The model under review builds one solid part; all positions refer to its coordinate system, in mm. A direction names the side the tool comes from. Round coordinates to 2 decimals unless told otherwise and drop trailing zeros. Loops run counter-clockwise (first coordinate to the right, second up) from the corner with the lowest first, then second, coordinate; pieces in that order, holes last. Notation, with made-up numbers: (74.25, -17.75) -> (94.25, -17.75) arc R20 ccw to (94.25, 21.25) -> close; hole circle Ø10 at (-1, -31.75). An arc over 180 degrees is marked (long way). Use a Markdown table: item, result. Add a question column.
1) Insertion check: pin 1 (1 mm diameter, centred on y = 5.5, z = -20, fed in from +X); pin 2 (4 mm diameter, centred on x = 8, y = 5.5, fed in from +Z); pin 3 (2.5 mm diameter, centred on x = -14.5, y = 4.5, fed in from -Z). Each pin has a flat end and moves straight along its axis. Give the tip position at first contact, or say it passes through.
2) Consider section A-A on x = 56. Give the boundary of the cut face in (y, z).
3) Mouldability with a two-part tool opening along Z and no side actions: class faces 4 (the flat face through (-17, 5, -15.155)), 5 (the flat face through (59, 5, -12.155)), 6 (the flat face through (59.8, 4.7, -6.155)), 7 (the cylindrical face through (-9.105, 5.137, 3.965)) as released by +Z, released by -Z, zero draft, split by the parting line, or undercut.
4) For faces 1 (the flat face through (53.686, 5, -9)), 2 (the flat face through (-23.899, 5, -9)), 3 (the flat face through (-17, 7.51, -9)), list the 3-axis set-ups (+Z, -Z, +X, -X, +Y, -Y) from which the entire face can be reached by the end or side of a thin tool; tool diameter is ignored.
5) Consider section B-B on z = -14. Give the boundary of the cut face in (x, y) (3 decimals).
6) Consider section C-C on x = 28. Give the boundary of the cut face in (y, z).
7) Wall thickness on probe 1 along Y at (x, z) = (-17.5, -5); probe 2 along Z at (x, y) = (-14, 6); probe 3 along X at (y, z) = (5.25, -11): over which ranges is each line inside the solid? List them lowest first.
8) Consider section D-D on x = -14. Give the boundary of the cut face in (y, z).
Autodesk Inventor part; units mm, degrees
ref_plane "Work Plane1" through (67.1008, 0, -24.4554) normal (0, 0, 1) x (-1, 0, 0)
ref_plane "Work Plane2" through (-11.8992, 0, -24.4554) normal (1, 0, 0) x (0, 0, 1)
ref_plane "YZ Plane" through (0, 0, 0) normal (1, 0, 0) x (0, 1, 0)
sketch "Sketch1" plane through (0, 0, 0) normal (0, 1, 0) x (-1, 0, 0)
  line L0 (11.8992, 6.1446) -> (-67.1008, 6.1446)
  line L1 (-67.1008, 6.1446) -> (-67.1008, -24.4554)
  line L2 (-67.1008, -24.4554) -> (11.8992, -24.4554)
  line L3 (11.8992, -24.4554) -> (11.8992, 6.1446)
  point P0 (0, 0)
  dimension "d0" = 79
  dimension "d1" = 30.6
extrude "Extrusion1" add sketch "Sketch1" along normal blind 9.51
sketch "Sketch3" plane through (-11.8992, 0, -24.4554) normal (-1, 0, 0) x (0, 0, 1)
  line L0 (0, 9.51) -> (30.6, 9.51)
  line L1 (15.3, 9.51) -> (0.75, 9.51)
  line L2 (30.6, 9.51) -> (0, 9.51)
  line L3 (0.75, 9.51) -> (29.85, 9.51)
  line L4 (30.6, 0) -> (30.6, 9.51)
  line L5 (0, 0) -> (0, 9.51)
  line L6 (30.6, 0) -> (0, 0)
  line L7 (30.6, 0) -> (29.85, 9.51)
  line L8 (0, 0) -> (0.75, 9.51)
  point P0 (24.4554, 0)
  dimension "d4" = 14.55
  dimension "d5" = 29.1
extrude "Extrusion2" cut sketch "Sketch3" against normal through all contours L0 L8 L5 | L7 L0 L4
ref_plane "Work Plane1" through (67.1008, 0, -24.4554) normal (0, 0, 1) x (-1, 0, 0)
sketch "Sketch5" plane through (67.1008, 0, -24.4554) normal (0, 0, 1) x (-1, 0, 0)
  line L0 (0, -9.51) -> (79, -9.51)
  line L1 (79, -9.51) -> (79, 0)
  line L2 (0, 0) -> (0, -9.51)
  line L3 (79, -9.51) -> (0, -9.51)
  line L4 (39.5, -9.51) -> (77, -9.51)
  line L5 (77, -9.51) -> (79, 0)
  line L6 (79, 0) -> (79, -9.51)
  line L7 (79, -9.51) -> (79, 0)
  line L8 (39.5, -9.51) -> (2, -9.51)
  line L9 (0, -9.51) -> (0, 0)
  line L10 (2, -9.51) -> (0, 0)
  line L11 (0, 0) -> (0, -9.51)
  line L12 (0, -9.51) -> (2, -9.51)
  point P0 (67.1008, 0)
  dimension "d11" = 37.5
  dimension "d12" = 37.5
extrude "Extrusion3" cut sketch "Sketch5" along normal through all
ref_plane "Work Plane2" through (-11.8992, 0, -24.4554) normal (1, 0, 0) x (0, 0, 1)
sketch "Sketch7" plane through (-11.8992, 0, -24.4554) normal (1, 0, 0) x (0, 0, 1)
  line L0 (0, 0) -> (30.6, 0)
  line L1 (0.75, -9.51) -> (29.85, -9.51)
  line L2 (29.85, -9.51) -> (30.6, 0)
  line L3 (0, 0) -> (0.75, -9.51)
  line L4 (15.3, 0) -> (15.3, -9.51)
  line L5 (28.0015, -7.51) -> (2.5985, -7.51)
  line L6 (2.5985, -7.51) -> (2.1639, -2)
  line L7 (2.1639, -2) -> (28.4361, -2)
  line L8 (28.4361, -2) -> (28.0015, -7.51)
  line L9 (27.3541, -3) -> (3.2459, -3)
  line L10 (3.2459, -3) -> (3.5227, -6.51)
  line L11 (3.5227, -6.51) -> (27.0773, -6.51)
  line L12 (27.0773, -6.51) -> (27.3541, -3)
  line L13 (15.3, -3) -> (15.3, -7.51)
  line L14 (21.3, -3) -> (9.3, -3)
  line L15 (9.3, -3) -> (9.3, -7.51)
  line L16 (9.3, -7.51) -> (21.3, -7.51)
  line L17 (21.3, -7.51) -> (21.3, -3)
  line L18 (21.3, -3) -> (9.3, -7.51) construction
  line L19 (9.3, -3) -> (21.3, -7.51) construction
  point P0 (24.4554, 0)
  point P1 (15.3, -5.255)
  dimension "d16" = 2
  dimension "d17" = 3
  dimension "d18" = 12
extrude "Extrusion4" add sketch "Sketch7" along normal blind 10 contours L9 L17 L11 L4 | L4 L11 L15 L9 | L5 L15 L11 L4 | L4 L11 L17 L5
sketch "Sketch8" plane through (-11.8992, 0, -24.4554) normal (-1, 0, 0) x (0, 0, 1)
  line L0 (9.3, 7.51) -> (21.3, 7.51)
  line L1 (9.3, 3) -> (9.3, 7.51)
  line L2 (21.3, 3) -> (9.3, 3)
  line L3 (21.3, 7.51) -> (21.3, 3)
  point P0 (24.4554, 0)
extrude "Extrusion5" add sketch "Sketch8" along normal blind 12
sketch "Sketch9" plane through (67.1008, 0, -24.4554) normal (0, 0, 1) x (-1, 0, 0)
  line L0 (0, 0) -> (79, 0)
  line L1 (2, -9.51) -> (77, -9.51)
  line L2 (0, -4.755) -> (79, -4.755)
  line L3 (2, -9.51) -> (0, 0)
  line L4 (4.9287, 0) -> (79, 0)
  line L5 (1.0143, -4.8232) -> (2, -9.51)
  arc A0 (4.9287, 0) -> (1.0143, -4.8232) centre (4.9287, -4) ccw
  point P0 (67.1008, 0)
  point P1 (4.9287, 0)
  dimension "d23" = 9.51
  dimension "d24" = 4.755
  dimension "d25" = 4
extrude "Extrusion6" cut sketch "Sketch9" along normal through all
sketch "Sketch10" plane through (67.1008, 0, -24.4554) normal (0, 0, 1) x (-1, 0, 0)
  line L0 (4.9287, 0) -> (79, 0)
  line L1 (2, -9.51) -> (77, -9.51)
  line L2 (4.9287, -4.755) -> (79, -4.755)
  line L3 (2, -9.51) -> (1.0143, -4.8232)
  circle A0 centre (5.859, -4.755) radius 4.755
  circle A1 centre (5.859, -4.755) radius 1.25
  point P0 (67.1008, 0)
  dimension "d28" = 9.51
  dimension "d29" = 4.755
  dimension "d31" = 2.5
extrude "Extrusion7" cut sketch "Sketch10" along normal through all contours A1
sketch "Sketch11" plane through (0, 0, 0) normal (0, -1, 0) x (1, 0, 0)
  line L0 (-11.8992, 6.1446) -> (62.1721, 6.1446)
  line L1 (62.1721, -24.4554) -> (-11.8992, -24.4554)
  line L2 (-11.8992, -6.1554) -> (62.1721, -6.1554)
  line L3 (62.1721, -12.1554) -> (-11.8992, -12.1554)
  line L4 (25.1364, -6.1554) -> (66.0864, -6.1554)
  line L5 (66.0864, 5.7642) -> (66.0864, -24.075)
  line L6 (25.1364, -12.1554) -> (66.0864, -12.1554)
  line L7 (65.1008, 5.3946) -> (65.1008, -23.7054)
  line L8 (66.0864, -6.1554) -> (53.6864, -6.1554)
  line L9 (53.6864, -6.1554) -> (53.6864, -12.1554)
  line L10 (66.1721, 5.8291) -> (66.1721, -24.1399)
  line L11 (66.0864, -6.1554) -> (66.1721, -6.1554)
  line L12 (66.0864, -12.1554) -> (66.1721, -12.1554)
  point P0 (0, 0)
  dimension "d34" = 12.3
  dimension "d35" = 12.3
  dimension "d36" = 12.4
extrude "Extrusion8" cut sketch "Sketch11" against normal through all
fillet "Fillet1" radius 6 2 edges at (-10.8992, 4.755, 5.7696) (-10.8992, 4.755, -24.0804)
ref_plane "Work Plane3" through (65.1008, 9.51, -16.8054) normal (0.205803, -0.9785934, 0) x (0, 0, -1)
properties part number "ArcherT4U_USB"
Result set:
| question | item | result |
|---|---|---|
| 1 | pin 1 | x = 66.05 |
| 1 | pin 2 | z = 5.87 |
| 1 | pin 3 | z = -15.16 |
| 2 | outline | (0, -24.46) -> (9.51, -23.71) -> (9.51, -12.16) -> (0, -12.16) -> close; (0, -6.16) -> (9.51, -6.16) -> (9.51, 5.39) -> (0, 6.14) -> close |
| 3 | face 4 | released by -Z |
| 3 | face 5 | undercut |
| 3 | face 6 | undercut |
| 3 | face 7 | released by +Z |
| 4 | face 1 | +X, +Y, -Y |
| 4 | face 2 | +Z, -Z, -X, +Y, -Y |
| 4 | face 3 | +Z, -Z, -X, +Y |
| 5 | outline | (-23.899, 3) -> (-11.268, 3) -> (-11.899, 0) -> (62.172, 0) arc R4 ccw to (66.1, 4.755) -> (65.101, 9.51) -> (-9.899, 9.51) -> (-10.32, 7.51) -> (-23.899, 7.51) -> close; hole circle Ø2.5 at (61.242, 4.755) |
| 6 | outline | (0, -24.46) -> (9.51, -23.71) -> (9.51, 5.39) -> (0, 6.14) -> close |
| 7 | probe 1 | 3 to 7.51 |
| 7 | probe 2 | -15.16 to -3.16 |
| 7 | probe 3 | -23.9 to 53.69 |
| 8 | outline | (3, -15.16) -> (7.51, -15.16) -> (7.51, -3.16) -> (3, -3.16) -> close |
